Can you work these out from the model? Positions are in its coordinate system, mm. Face numbers are marked on the shaded views. A direction names the side the tool comes from. Give positions to 0.01 mm unless a question says otherwise; leave off trailing zeros. Order: outer loops, then holes, each group sorted by start corner. A loop starts at its lowest first (then second) coordinate and runs counter-clockwise, first axis right, second up. Notation, with made-up numbers: (89.25, 1) -> (132.25, 1) arc R9 ccw to (132.25, 15) -> close; hole circle Ø5 at (22.5, 23.5). An arc over 180 degrees is marked (long way). Answer as a JSON object with one key per item and string values.
```python
from build123d import *

# Parameters (mm, degrees)
SKETCH1_W           = 102.2
SKETCH1_H           = 92.45
SKETCH1_R           = 1.6
BOSS_EXTRUDE1_DEPTH = 6
SKETCH2_W           = 138.2
SKETCH2_H           = 92.45
SKETCH2_R           = 2.5
BOSS_EXTRUDE2_DEPTH = 3.2
FILLET1_R           = 6
FILLET2_R           = 5
FILLET3_R           = 5


with BuildPart() as part:
    # Sketch1 → Boss-Extrude1 (new body)
    with BuildSketch(Plane.XY):
        with Locations((51.1, 46.225)):
            Rectangle(SKETCH1_W, SKETCH1_H)
        with BuildLine():
            Line((94.706674091, 2.5), (7.493325909, 2.5))
            ThreePointArc((7.493325909, 2.5), (7.045584412, 7.045584412), (2.5, 7.493325909))
            Line((2.5, 7.493325909), (2.5, 90.25))
            Line((2.5, 90.25), (99.7, 90.25))
            Line((99.7, 90.25), (99.7, 57.093325909))
            ThreePointArc((99.7, 57.093325909), (94.1, 54.1), (99.7, 51.106674091))
            Line((99.7, 51.106674091), (99.7, 7.493325909))
            ThreePointArc((99.7, 7.493325909), (95.154415588, 7.045584412), (94.706674091, 2.5))
        make_face(mode=Mode.SUBTRACT)
        with Locations((4.5, 4.5)):
            Circle(SKETCH1_R, mode=Mode.SUBTRACT)
        with Locations((97.7, 4.5)):
            Circle(SKETCH1_R, mode=Mode.SUBTRACT)
        with Locations((97.7, 54.1)):
            Circle(SKETCH1_R, mode=Mode.SUBTRACT)
    extrude(amount=BOSS_EXTRUDE1_DEPTH)

    # Sketch2 → Boss-Extrude2 (add)
    with BuildSketch(Plane(origin=(0, 0, 0), x_dir=(-1, 0, 0), z_dir=(0, 0, -1))):
        with Locations((-51.1, 46.225)):
            Rectangle(SKETCH2_W, SKETCH2_H)
        with Locations((-112.2, 84.45)):
            Circle(SKETCH2_R, mode=Mode.SUBTRACT)
        with Locations((-112.2, 8)):
            Circle(SKETCH2_R, mode=Mode.SUBTRACT)
        with Locations((10, 8)):
            Circle(SKETCH2_R, mode=Mode.SUBTRACT)
        with Locations((10, 84.45)):
            Circle(SKETCH2_R, mode=Mode.SUBTRACT)
    extrude(amount=BOSS_EXTRUDE2_DEPTH)

    # Fillet1
    fillet1_edges = [part.edges().sort_by_distance(p)[0] for p in [
        (120.2, 92.45, -1.6),
        (120.2, 0, -1.6),
        (-18, 0, -1.6),
        (-18, 92.45, -1.6),
    ]]
    fillet(fillet1_edges, radius=FILLET1_R)

    # Fillet2
    fillet2_edges = [part.edges().sort_by_distance(p)[0] for p in [
        (99.7, 51.106674091, 3),
        (99.7, 57.093325909, 3),
    ]]
    fillet(fillet2_edges, radius=FILLET2_R)

    # Fillet3
    fillet3_edges = [part.edges().sort_by_distance(p)[0] for p in [
        (7.493325909, 2.5, 3),
        (94.706674091, 2.5, 3),
        (99.7, 7.493325909, 3),
        (2.5, 7.493325909, 3),
    ]]
    fillet(fillet3_edges, radius=FILLET3_R)


solid = part.part
```
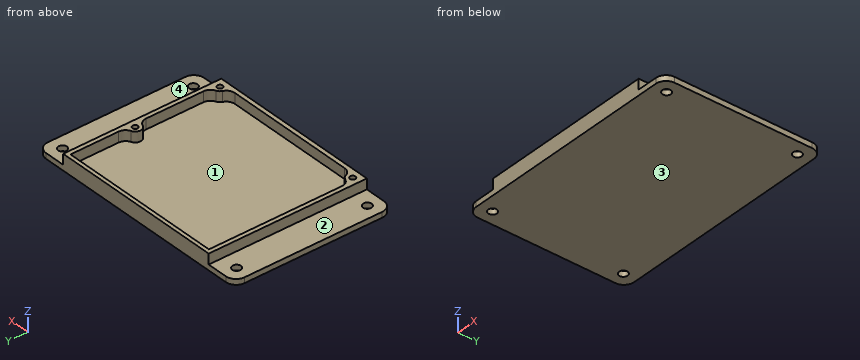
1. If we section it at B-B on x = 112.2: Please give me the cut outline in (y, z), then the cut area to 3 significant figures.
Worked answers:
{"outline": "(0, -3.2) -> (5.5, -3.2) -> (5.5, 0) -> (0, 0) -> close; (10.5, -3.2) -> (81.95, -3.2) -> (81.95, 0) -> (10.5, 0) -> close; (86.95, -3.2) -> (92.45, -3.2) -> (92.45, 0) -> (86.95, 0) -> close", "area": "264 mm²"}
2. If we mould it in two halves opening along Y, with no side actions, what happens to the marked faces 1 and 2? For each: +Y half, -Y half, draft (parallel to the pull), parting line (faces both ways), or undercut.
Worked answers:
{"face 1": "undercut", "face 2": "draft"}
3. Please list where these lines run through material, in increasing order: L1, parallel to Y at x = 97.7, z = 3.45; L2, parallel to X at y = 76, z = 2.5; L3, parallel to Y at x = 61.5, z = 2.5.
Worked answers:
{"L1": "0 to 2.9, 6.1 to 8.56, 50.04 to 52.5, 55.7 to 58.16, 90.25 to 92.45", "L2": "0 to 2.5, 99.7 to 102.2", "L3": "0 to 2.5, 90.25 to 92.45"}
4. If we section it at A-A on y = 84.45: Please give me the cut outline in (x, z), then the cut area to 3 significant figures.
Worked answers:
{"outline": "(-18, -3.2) -> (-12.5, -3.2) -> (-12.5, 0) -> (-18, 0) -> close; (-7.5, -3.2) -> (109.7, -3.2) -> (109.7, 0) -> (102.2, 0) -> (102.2, 6) -> (99.7, 6) -> (99.7, 0) -> (2.5, 0) -> (2.5, 6) -> (0, 6) -> (0, 0) -> (-7.5, 0) -> close; (114.7, -3.2) -> (120.2, -3.2) -> (120.2, 0) -> (114.7, 0) -> close", "area": "440 mm²"}
5. If we section it at C-C on z = 1.5: Please give me the cut outline in (x, y), then the cut area to 3 significant figures.
Worked answers:
{"outline": "(0, 0) -> (102.2, 0) -> (102.2, 92.45) -> (0, 92.45) -> close; hole (2.5, 12.56) arc R5 ccw to (5.76, 7.87) arc R3.6 cw to (7.87, 5.76) arc R5 ccw to (12.56, 2.5) -> (89.64, 2.5) arc R5 ccw to (94.33, 5.76) arc R3.6 cw to (96.44, 7.87) arc R5 ccw to (99.7, 12.56) -> (99.7, 46.04) arc R5 ccw to (96.44, 50.73) arc R3.6 cw to (96.44, 57.47) arc R5 ccw to (99.7, 62.16) -> (99.7, 90.25) -> (2.5, 90.25) -> close; hole circle Ø3.2 at (4.5, 4.5); hole circle Ø3.2 at (97.7, 4.5); hole circle Ø3.2 at (97.7, 54.1)", "area": "1,010 mm²"}
6. If we section it at D-D on y = 54.1: Please give me the cut outline in (x, z), then the cut area to 3 significant figures.
Worked answers:
{"outline": "(-18, -3.2) -> (120.2, -3.2) -> (120.2, 0) -> (102.2, 0) -> (102.2, 6) -> (99.3, 6) -> (99.3, 0) -> (96.1, 0) -> (96.1, 6) -> (94.1, 6) -> (94.1, 0) -> (2.5, 0) -> (2.5, 6) -> (0, 6) -> (0, 0) -> (-18, 0) -> close", "area": "487 mm²"}
7. For the marked faces 3 and 4, which set-ups out of +Z, -Z, +X, -X, +Y, -Y let a thin tool reach every point of the face, with its end or its side?
Worked answers:
{"face 3": "-Z, +X, -X, +Y, -Y", "face 4": "+Z, +X, +Y, -Y"}
8. Will these pins go through, and if not, where does the flat tip stop? pin 1 Ø6 at (x, y) = (-10, 84.45) entering from +Z; pin 2 Ø5 at (y, z) = (55.5, 4.5) entering from +X; pin 3 Ø2 at (y, z) = (65, 4) entering from -X; pin 4 Ø3 at (x, y) = (112.2, 8) entering from -Z.
Worked answers:
{"pin 1": "z = 0", "pin 2": "x = 102.2", "pin 3": "x = 0", "pin 4": "through"}
